```python
from build123d import *

# Parameters (mm, degrees)
EXTRUDE_1_DEPTH     = 10
SKETCH_2_R          = 2
CUT_EXTRUDE_1_DEPTH = 10


with BuildPart() as part:
    # 草图1 → 凸台-拉伸1 (new body)
    with BuildSketch(Plane(origin=(0, 0, 0), x_dir=(1, 0, 0), z_dir=(0, 1, 0))):
        with BuildLine():
            Line((-39, 0.885049463), (-25.931575126, 0.885049463))
            ThreePointArc((-25.931575126, 0.885049463), (-25.250583901, 1.152757888), (-24.934206852, 1.81254756))
            ThreePointArc((-24.934206852, 1.81254756), (-23.860011776, 7.463232411), (-21.522796165, 12.718853928))
            Line((-21.522796165, 12.718853928), (-26.30015626, 12.718853928))
            Line((-26.30015626, 12.718853928), (-25.721769935, 13.718853928))
            Line((-25.721769935, 13.718853928), (-20.899594419, 13.718853928))
            ThreePointArc((-20.899594419, 13.718853928), (-19.738763969, 15.342137953), (-18.45215564, 16.867659952))
            Line((-18.45215564, 16.867659952), (-23.900543591, 16.867659952))
            Line((-23.900543591, 16.867659952), (-23.245613592, 18))
            Line((-23.245613592, 18), (-17.349351573, 18))
            ThreePointArc((-17.349351573, 18), (0, 25), (17.349351573, 18))
            Line((17.349351573, 18), (23.245613592, 18))
            Line((23.245613592, 18), (23.900543591, 16.867659952))
            Line((23.900543591, 16.867659952), (18.45215564, 16.867659952))
            ThreePointArc((18.45215564, 16.867659952), (19.738763969, 15.342137953), (20.899594419, 13.718853928))
            Line((20.899594419, 13.718853928), (25.721769935, 13.718853928))
            Line((25.721769935, 13.718853928), (26.30015626, 12.718853928))
            Line((26.30015626, 12.718853928), (21.522796165, 12.718853928))
            ThreePointArc((21.522796165, 12.718853928), (23.865801222, 7.44469825), (24.936992355, 1.773812925))
            ThreePointArc((24.936992355, 1.773812925), (25.252344114, 1.113532593), (25.932918663, 0.844766649))
            Line((25.932918663, 0.844766649), (39.00132777, 0.82446634))
            ThreePointArc((39.00132777, 0.82446634), (39.708888674, 1.116260796), (40.002879949, 1.822911748))
            Line((40.002879949, 1.822911748), (40.00771867, 4.937858527))
            Line((40.00771867, 4.937858527), (34.656523892, 4.946171008))
            ThreePointArc((34.656523892, 4.946171008), (32.159247749, 5.618953494), (30.332223376, 7.44952891))
            Line((30.332223376, 7.44952891), (26.1380565, 14.727086916))
            Line((26.1380565, 14.727086916), (21.201804646, 14.727086916))
            Line((21.201804646, 14.727086916), (20.426778105, 15.735319903))
            Line((20.426778105, 15.735319903), (25.55547359, 15.735319903))
            Line((25.55547359, 15.735319903), (23.669823804, 18.999997983))
            Line((23.669823804, 18.999997983), (17.250673347, 18.999997983))
            Line((17.250673347, 18.999997983), (16.002596538, 19.999997983))
            Line((16.002596538, 19.999997983), (23.091437479, 19.999997983))
            Line((23.091437479, 19.999997983), (18.787180185, 27.482043412))
            ThreePointArc((18.787180185, 27.482043412), (16.958217309, 29.315990717), (14.457053173, 29.98878035))
            Line((14.457053173, 29.98878035), (-14.410451579, 30.011201553))
            ThreePointArc((-14.410451579, 30.011201553), (-16.910971111, 29.343270507), (-18.742519025, 27.514565487))
            Line((-18.742519025, 27.514565487), (-23.088840941, 20))
            Line((-23.088840941, 20), (-16, 20))
            Line((-16, 20), (-17.248076809, 19))
            Line((-17.248076809, 19), (-23.667227267, 19))
            Line((-23.667227267, 19), (-25.55547359, 15.735319903))
            Line((-25.55547359, 15.735319903), (-20.426778105, 15.735319903))
            Line((-20.426778105, 15.735319903), (-21.201804646, 14.727086916))
            Line((-21.201804646, 14.727086916), (-26.138621763, 14.727086916))
            Line((-26.138621763, 14.727086916), (-30.320614786, 7.496637574))
            ThreePointArc((-30.320614786, 7.496637574), (-32.150480545, 5.668902441), (-34.648798766, 5))
            Line((-34.648798766, 5), (-39, 5))
            ThreePointArc((-39, 5), (-39.707106781, 4.707106781), (-40, 4))
            Line((-40, 4), (-40, 1.885049463))
            ThreePointArc((-40, 1.885049463), (-39.707106781, 1.177942682), (-39, 0.885049463))
        make_face()
    extrude(amount=EXTRUDE_1_DEPTH)

    # 草图2 → 切除-拉伸1 (cut)
    with BuildSketch(Plane.XY):
        with Locations((35, 5)):
            Circle(SKETCH_2_R)
        with Locations(Location((-35, 5, 0), (0, 0, 79.886387813))):
            Circle(SKETCH_2_R)
    extrude(amount=-CUT_EXTRUDE_1_DEPTH, mode=Mode.SUBTRACT)


solid = part.part
```
The model under review builds one solid part; all positions refer to its coordinate system, in mm. A direction names the side the tool comes from. Coordinates: 2 decimals unless noted, no trailing zeros. Write each loop counter-clockwise with the first axis right and the second up, starting at its lowest first coordinate (ties: lowest second). Pieces come first, ordered by that corner, then holes.
1) To check wall thickness, follow probe 1 along X at (y, z) = (5, -1.75); probe 2 along Y at (x, z) = (-35, -4.25); probe 3 along X at (y, z) = (5, -3.75). State the ranges of each line that lie inside material, in increasing order.
2) We need section B-B on y = 5. Count the separate pieces of the cut face and the enclosed holes in it, then the cut area to 3 significant figures.
3) Machinability: for faces 1 (the face through (-20, 5, -18)), 2 (the face through (21, 5, -19)), 3 (the face through (23.842, 4.93, -7.522)), 4 (the face through (-3, 10, -25)), 5 (the face through (-32.6, 4.9, -0.885)), which of the approach directions +Z, -Z, +X, -X, +Y, -Y give a long, thin tool a straight path to every point of the face, cutting with its end or side? Answer none if there is none.
4) The part is to be moulded in two halves that separate along Z. For faces 6 (the face through (-28.2, 4.93, -11.16)), 7 (the face through (33, 5, -3)), 8 (the face through (23, 5, -13.719)), say which applies: pulls with the +Z half, pulls with the -Z half, needs draft (parallel to the pull), parting line crosses it, or undercut.
5) We need section D-D on x = -29.5. State the section outline as (y, z) points, then the cut area to 3 significant figures.
6) We need section C-C on z = -21.5. State the section outline as (x, y) points, then the cut area to 3 significant figures.
7) We need section A-A on z = -11.5. State the section outline as (x, y) points, then the cut area to 3 significant figures.
8) Clearance check with flat-ended pins moving along their axes: pin 1 Ø1.3 at (x, y) = (-37, 4) entering from -Z; pin 2 Ø4 at (x, y) = (23.5, 6) entering from -Z; pin 3 Ø4 at (x, y) = (-24, 6.5) entering from +Z. State where each tip first meets the part, or that it passes through.
Answer list:
1. probe 1: x = -39.99 to -37, -33 to -24.94, 24.94 to 33, 37 to 40
1. probe 2: y = 0 to 3, 7 to 10
1. probe 3: x = -40 to -37, -33 to -24.72, 24.72 to 33, 37 to 40.01
2. separate pieces: 3
2. enclosed holes: 0
2. area: 539 mm2
3. face 1: +Y, -Y
3. face 2: +X, +Y, -Y
3. face 3: +Z, +Y, -Y
3. face 4: +Z, -Z, +X, -X, +Y
3. face 5: +Z, -X, +Y, -Y
4. face 6: pulls with the -Z half
4. face 7: needs draft
4. face 8: undercut
5. outline: (0, -8.92) - (10, -8.92) - (10, -0.89) - (0, -0.89) - close
5. area: 80.3 mm2
6. outline: (-22.22, 0) - (-12.76, 0) - (-12.76, 10) - (-22.22, 10) - close; (12.76, 0) - (22.23, 0) - (22.23, 10) - (12.76, 10) - close
6. area: 189 mm2
7. outline: (-28.01, 0) - (-22.2, 0) - (-22.2, 10) - (-28.01, 10) - close; (22.2, 0) - (28, 0) - (28, 10) - (22.2, 10) - close
7. area: 116 mm2
8. pin 1: stops at z = -5
8. pin 2: stops at z = -22.77
8. pin 3: stops at z = -0.89
